Model file for the job. Use its own axes, mm. Face numbers are marked on the shaded views. A direction names the side the tool comes from. Round coordinates to 2 decimals unless told otherwise and drop trailing zeros. Order: outer loops, then holes, each group sorted by start corner. A loop starts at its lowest first (then second) coordinate and runs counter-clockwise, first axis right, second up. Notation, with made-up numbers: (-31.75, -39) - (4.25, -39) arc R31 cw to (4.25, -13) - close; hole circle Ø2 at (-36, 59). An arc over 180 degrees is marked (long way). Put each result on its own line as item: value. Start each with the question number.
Item 1: Which spindle directions (+Z, -Z, +X, -X, +Y, -Y) get a long thin tool onto all of the face, cutting with end or side? Do the marked faces 4 and 5. Say none if no direction does.
Item 2: Probe probe 1 along Y at (x, z) = (15, 0); probe 2 along Y at (x, z) = (9.25, 2); probe 3 along Y at (x, z) = (20.2, 0). List the from-to ranges inside material, lowest first.
Item 3: Saw through at B-B on y = 39. List the corners of the cut face in (x, z), plus the area to 3 significant figures.
Item 4: Pin check, flat tips, straight feed: pin 1 Ø4 at (y, z) = (0, -39) entering from -X; pin 2 Ø6 at (y, z) = (0, 39) entering from -X; pin 3 Ø3 at (x, z) = (12, 18) entering from -Y; pin 4 Ø1 at (x, y) = (6, 18.5) entering from +Z. Stop position of each tip, or through.
Item 5: Saw through at D-D on x = 16.75. List the corners of the cut face in (y, z), plus the area to 3 significant figures.
Item 6: Saw through at C-C on z = 11. List the corners of the cut face in (x, y), plus the area to 3 significant figures.
Item 7: Mould opens along Y. For the marked faces 1, 2 and 3 say: pulls with the +Y half, pulls with the -Y half, needs draft (parallel to the pull), parting line crosses it, or undercut.
Item 8: Saw through at A-A on z = 0. List the corners of the cut face in (x, y), plus the area to 3 significant figures.
```python
from build123d import *

# Parameters (mm, degrees)
SKETCH_1_R          = 44
SKETCH_1_R_2        = 31
EXTRUDE_1_DEPTH     = 17.9
SKETCH_2_R          = 2.5
CUT_EXTRUDE_1_DEPTH = 17.9
SKETCH_3_R          = 34
SKETCH_3_R_2        = 16
EXTRUDE_2_DEPTH     = 5


with BuildPart() as part:
    # 草图1 → 凸台-拉伸1 (new body)
    with BuildSketch(Plane(origin=(0, 0, 0), x_dir=(0, 0, -1), z_dir=(1, 0, 0))):
        with Locations(Location((0, 0, 0), (0, 0, 180))):
            Circle(SKETCH_1_R)
        with Locations(Location((0, 0, 0), (0, 0, 180))):
            Circle(SKETCH_1_R_2, mode=Mode.SUBTRACT)
    extrude(amount=EXTRUDE_1_DEPTH)

    # 草图2 → 切除-拉伸1 (cut)
    with BuildSketch(Plane(origin=(17.9, 0, 0), x_dir=(0, 0, -1), z_dir=(1, 0, 0))):
        with Locations((0, 39)):
            Circle(SKETCH_2_R)
        with Locations((39, 0)):
            Circle(SKETCH_2_R)
        with Locations((0, -39)):
            Circle(SKETCH_2_R)
        with Locations((-39, 0)):
            Circle(SKETCH_2_R)
    extrude(amount=-CUT_EXTRUDE_1_DEPTH, mode=Mode.SUBTRACT)

    # 草图3 → 凸台-拉伸2 (add)
    with BuildSketch(Plane(origin=(17.9, 0, 0), x_dir=(0, 0, -1), z_dir=(1, 0, 0))):
        Circle(SKETCH_3_R)
        Circle(SKETCH_3_R_2, mode=Mode.SUBTRACT)
    extrude(amount=EXTRUDE_2_DEPTH)


solid = part.part
```
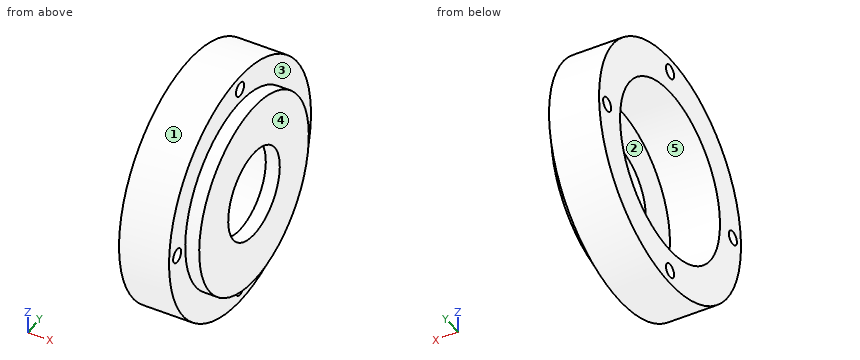
Results found:
1. face 4: +Z, -Z, +X, +Y, -Y
1. face 5: -X
2. probe 1: y = -44 to -41.5, -36.5 to -31, 31 to 36.5, 41.5 to 44
2. probe 2: y = -43.95 to -40.5, -37.5 to -30.94, 30.94 to 37.5, 40.5 to 43.95
2. probe 3: y = -34 to -16, 16 to 34
3. outline: (0, -20.37) - (17.9, -20.37) - (17.9, -2.5) - (0, -2.5) - close; (0, 2.5) - (17.9, 2.5) - (17.9, 20.37) - (0, 20.37) - close
3. area: 640 mm²
4. pin 1: passes through
4. pin 2: stops at x = 0
4. pin 3: stops at y = -40.79
4. pin 4: stops at z = 40.15
5. outline: circle Ø88 at (0, 0); hole circle Ø5 at (-39, 0); hole circle Ø62 at (0, 0); hole circle Ø5 at (0, -39); hole circle Ø5 at (0, 39); hole circle Ø5 at (39, 0)
5. area: 2,980 mm²
6. outline: (0, -42.6) - (17.9, -42.6) - (17.9, -32.17) - (22.9, -32.17) - (22.9, -11.62) - (17.9, -11.62) - (17.9, -28.98) - (0, -28.98) - close; (0, 28.98) - (17.9, 28.98) - (17.9, 11.62) - (22.9, 11.62) - (22.9, 32.17) - (17.9, 32.17) - (17.9, 42.6) - (0, 42.6) - close
6. area: 693 mm²
7. face 1: parting line crosses it
7. face 2: undercut
7. face 3: needs draft
8. outline: (0, -44) - (17.9, -44) - (17.9, -41.5) - (0, -41.5) - close; (0, -36.5) - (17.9, -36.5) - (17.9, -34) - (22.9, -34) - (22.9, -16) - (17.9, -16) - (17.9, -31) - (0, -31) - close; (0, 31) - (17.9, 31) - (17.9, 16) - (22.9, 16) - (22.9, 34) - (17.9, 34) - (17.9, 36.5) - (0, 36.5) - close; (0, 41.5) - (17.9, 41.5) - (17.9, 44) - (0, 44) - close
8. area: 466 mm²
